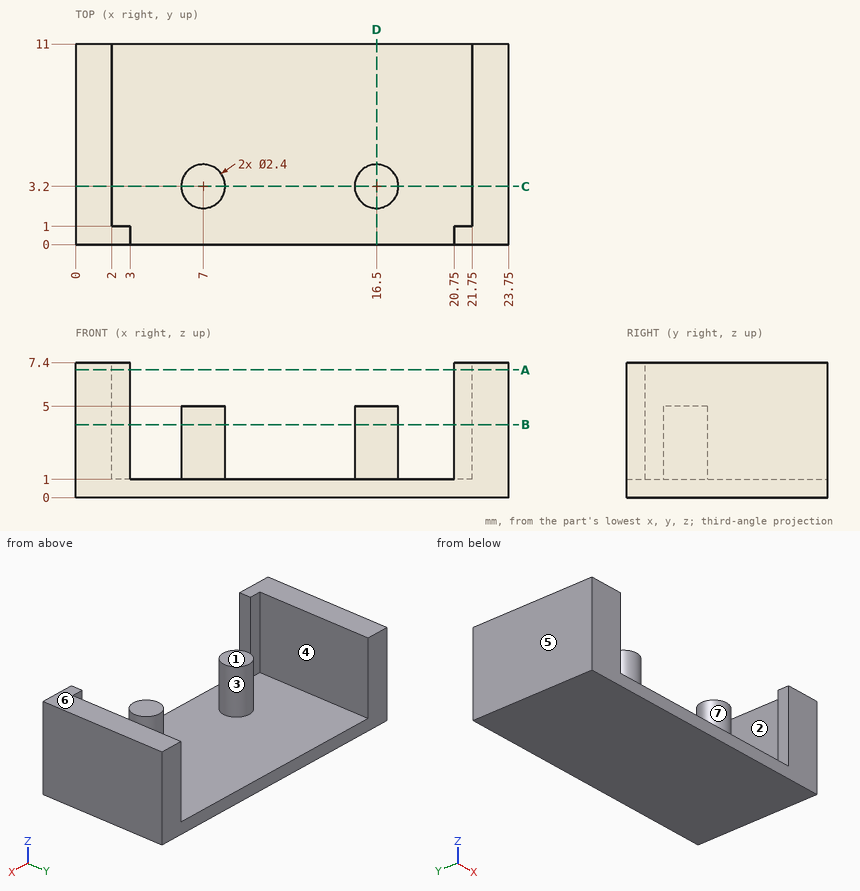
Geometry check sheet. Reference: drawing and pictorial views, mm from the part's lowest x, y, z. A direction names the side the tool comes from. Round coordinates to 2 decimals unless told otherwise and drop trailing zeros. Write each loop counter-clockwise with the first axis right and the second up, starting at its lowest first coordinate (ties: lowest second). Pieces come first, ordered by that corner, then holes.
Item 1: Material ranges on line 1 along X through (y, z) = (8.75, 2); line 2 along X through (y, z) = (3.5, 3); line 3 along Z through (x, y) = (13, 5.25), recorded low to high.
Determined:
line 1: x = 0 to 2, 21.75 to 23.75
line 2: x = 0 to 2, 5.84 to 8.16, 15.34 to 17.66, 21.75 to 23.75
line 3: z = 0 to 1
Item 2: Section check A-A (z = 7). Record the boundary of the cut face in (x, y).
Determined:
outline: (0, 0) - (3, 0) - (3, 1) - (2, 1) - (2, 11) - (0, 11) - close; (20.75, 0) - (23.75, 0) - (23.75, 11) - (21.75, 11) - (21.75, 1) - (20.75, 1) - close
Item 3: Section check B-B (z = 4). Record the boundary of the cut face in (x, y).
Determined:
outline: (0, 0) - (3, 0) - (3, 1) - (2, 1) - (2, 11) - (0, 11) - close; circle Ø2.4 at (7, 3.2); circle Ø2.4 at (16.5, 3.2); (20.75, 0) - (23.75, 0) - (23.75, 11) - (21.75, 11) - (21.75, 1) - (20.75, 1) - close
Item 4: Section check D-D (x = 16.5). Record the boundary of the cut face in (y, z), plus the area to 3 significant figures.
Determined:
outline: (0, 0) - (11, 0) - (11, 1) - (4.4, 1) - (4.4, 5) - (2, 5) - (2, 1) - (0, 1) - close
area: 20.6 mm2
Item 5: Access from +Z, -Z, +X, -X, +Y, -Y to the whole of each face (thin tool, end or side, straight path). Record for the marked faces 1, 2 and 3.
Determined:
face 1: +Z, +Y, -Y
face 2: +Z, +Y
face 3: +Z
Item 6: Mould release check, pull along X, two halves, no side actions. Record for the marked faces 4, 5, 6 and 7: +X half, -X half, draft (parallel to the pull), parting line (faces both ways), or undercut.
Determined:
face 4: undercut
face 5: -X half
face 6: draft
face 7: undercut
Item 7: Go/stop test with flat-tipped pins: pin 1 Ø0.5 at (y, z) = (0.5, 5) entering from -X; pin 2 Ø2 at (x, y) = (12.5, 7.5) entering from +Z; pin 3 Ø1.2 at (x, y) = (6.5, 3) entering from +Z; pin 4 Ø1.5 at (x, z) = (16.5, 6.5) entering from -Y. Record where each tip stops, or that it passes through.
Determined:
pin 1: stops at x = 0
pin 2: stops at z = 1
pin 3: stops at z = 5
pin 4: passes through
Item 8: Section check C-C (y = 3.2). Record the boundary of the cut face in (x, z).
Determined:
outline: (0, 0) - (23.75, 0) - (23.75, 7.4) - (21.75, 7.4) - (21.75, 1) - (17.7, 1) - (17.7, 5) - (15.3, 5) - (15.3, 1) - (8.2, 1) - (8.2, 5) - (5.8, 5) - (5.8, 1) - (2, 1) - (2, 7.4) - (0, 7.4) - close
